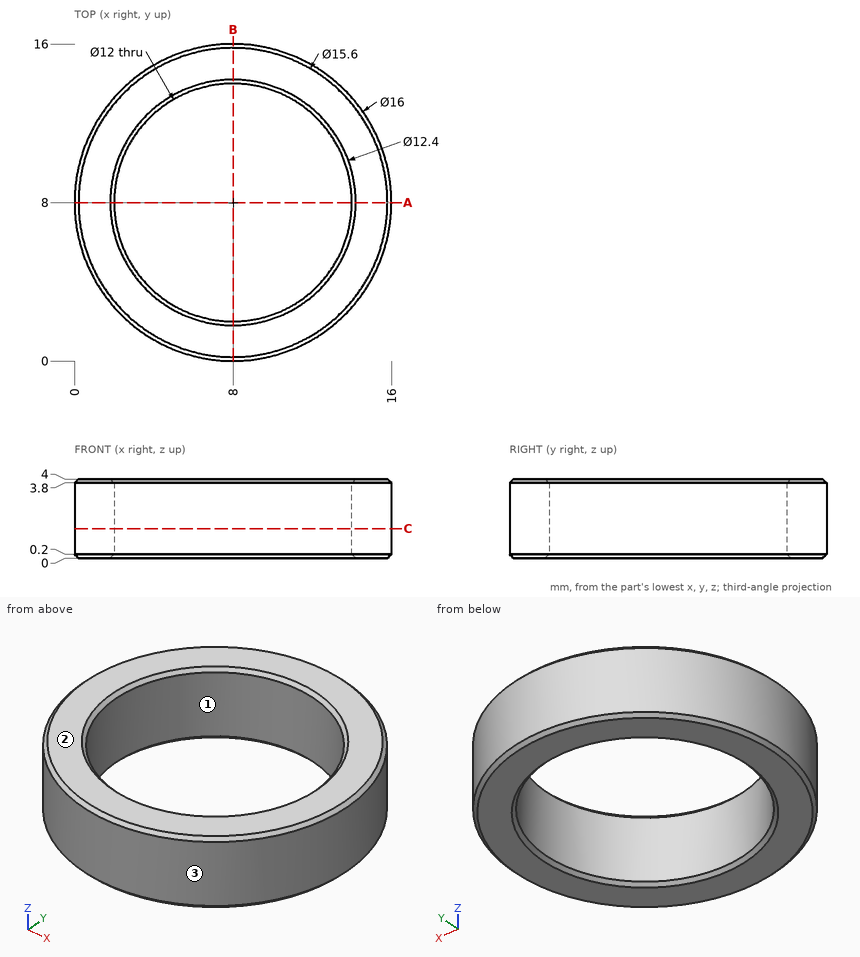
Design review of the part shown in the three views and the two pictorial views. Dimensions are in mm from the part's minimum x, y and z. Coordinates: 2 decimals unless noted, no trailing zeros. Order: outer loops, then holes, each group sorted by start corner. A loop starts at its lowest first (then second) coordinate and runs counter-clockwise, first axis right, second up. Notation, with made-up numbers: (18.5, 86.5) - (40.5, 86.5) arc R15 cw to (40.5, 94.5) - close; hole circle Ø4 at (-11.5, 2.5). An arc over 180 degrees is marked (long way). Answer as CSV lines item,"result". Start each with the question number.
1) To check wall thickness, follow line 1 along Y through (x, z) = (8, 2.6); line 2 along X through (y, z) = (12.5, 2.9); line 3 along Y through (x, z) = (10.25, 3.1). State the ranges of each line that lie inside material, in increasing order. Write a range as [from, to].
2) Add section C-C (z = 1.5). State the section outline as (x, y) points.
3) Add section A-A (y = 8). State the section outline as (x, z) points, then the cut area to 3 significant figures.
4) Insertion check: P1, Ø1.5, axis at x = 4, z = 3, coming from the +Y side; P2, Ø3, axis at x = 12, y = 7.5, coming from the -Z side; P3, Ø2, axis at x = 5.5, z = 2, coming from the +Y side. Each pin has a flat end and moves straight along its axis. Give the tip position at first contact, or say it passes through.
5) Draft analysis for pull direction Y (two halves, no side actions). For the marked faces 1, 2 and 3, state which applies: +Y half, -Y half, draft (parallel to the pull), parting line (faces both ways), or undercut.
Result:
1,line 1,"[0, 2], [14, 16]"
1,line 2,"[1.39, 4.03], [11.97, 14.61]"
1,line 3,"[0.32, 2.44], [13.56, 15.68]"
2,outline,"circle Ø16 at (8, 8); hole circle Ø12 at (8, 8)"
3,outline,"(0, 0.2) - (0.2, 0) - (1.8, 0) - (2, 0.2) - (2, 3.8) - (1.8, 4) - (0.2, 4) - (0, 3.8) - close; (14, 0.2) - (14.2, 0) - (15.8, 0) - (16, 0.2) - (16, 3.8) - (15.8, 4) - (14.2, 4) - (14, 3.8) - close"
3,area,"15.8 mm^2"
4,P1,"y = 15.31"
4,P2,"through"
4,P3,"y = 15.86"
5,face 1,"undercut"
5,face 2,"draft"
5,face 3,"parting line"
